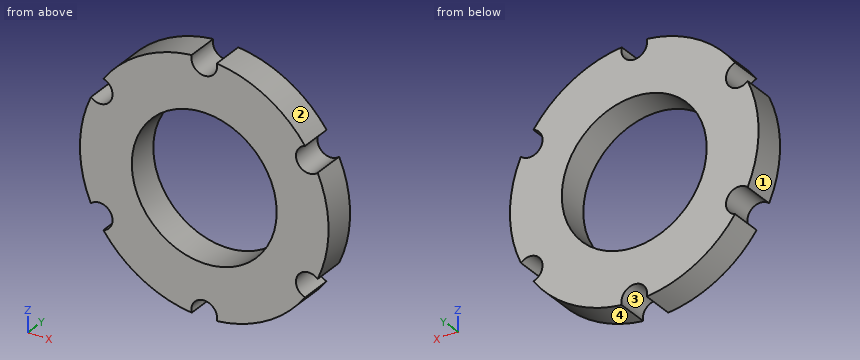
```python
from build123d import *

# Parameters (mm, degrees)
SKETCH1_R           = 30.861
SKETCH1_R_2         = 14.2875
BOSS_EXTRUDE1_DEPTH = 6.35
SKETCH2_R           = 2.54
CUT_EXTRUDE1_DEPTH  = 6.35
SKETCH3_R           = 30.861
SKETCH3_R_2         = 24.511
CUT_EXTRUDE2_DEPTH  = 45.103572894


with BuildPart() as part:
    # Sketch1 → Boss-Extrude1 (new body)
    with BuildSketch(Plane(origin=(0, 0, 0), x_dir=(1, 0, 0), z_dir=(0, 1, 0))):
        with Locations(Location((0, 0, 0), (0, 0, 270))):
            Circle(SKETCH1_R)
        with Locations(Location((0, 0, 0), (0, 0, 270))):
            Circle(SKETCH1_R_2, mode=Mode.SUBTRACT)
    extrude(amount=BOSS_EXTRUDE1_DEPTH)

    # Sketch2 → Cut-Extrude1 (cut)
    with BuildSketch(Plane(origin=(0, 6.35, 0), x_dir=(1, 0, 0), z_dir=(0, 1, 0))):
        with Locations(Location((0, 23.8125, 0), (0, 0, 270))):
            Circle(SKETCH2_R)
        with Locations(Location((0, -23.8125, 0), (0, 0, 270))):
            Circle(SKETCH2_R)
        with Locations(Location((20.622229928, 11.90625, 0), (0, 0, 270))):
            Circle(SKETCH2_R)
        with Locations(Location((20.622229928, -11.90625, 0), (0, 0, 270))):
            Circle(SKETCH2_R)
        with Locations(Location((-20.622229928, 11.90625, 0), (0, 0, 270))):
            Circle(SKETCH2_R)
        with Locations(Location((-20.622229928, -11.90625, 0), (0, 0, 270))):
            Circle(SKETCH2_R)
    extrude(amount=-CUT_EXTRUDE1_DEPTH, mode=Mode.SUBTRACT)

    # Sketch3 → Cut-Extrude2 (cut, through all)
    with BuildSketch(Plane(origin=(0, 6.35, 0), x_dir=(1, 0, 0), z_dir=(0, 1, 0))):
        Circle(SKETCH3_R)
        Circle(SKETCH3_R_2, mode=Mode.SUBTRACT)
    extrude(amount=-CUT_EXTRUDE2_DEPTH, mode=Mode.SUBTRACT)


solid = part.part
```
Input: part model. Units: mm. Frame: model coordinates. Face numbers are marked on the shaded views. Coordinates: 2 decimals unless noted, no trailing zeros. Loops run counter-clockwise (first coordinate to the right, second up) from the corner with the lowest first, then second, coordinate; pieces in that order, holes last.
Q1. Mould query, pull axis Z, two halves, no side actions, for the marked faces 1, 2, 3 and 4. Classes: +Z half, -Z half, draft (parallel to the pull), parting line (faces both ways), or undercut.
Results are:
face 1: parting line
face 2: +Z half
face 3: undercut
face 4: -Z half
Q2. Contact query for flat-ended pins moving along their axis: pin 1 (3 mm diameter, centred on y = 1.5, z = 18.5, fed in from +X); pin 2 (3 mm diameter, centred on y = 3.5, z = -11, fed in from -X); pin 3 (1.5 mm diameter, centred on x = -5, y = 4.5, fed in from +Z). Output: stop coordinate, or through.
Results are:
pin 1: stops at x = 17.66
pin 2: stops at x = -22.6
pin 3: stops at z = 24.14
Q3. Section C-C, the plane y = 1.25. Return the cut outline in (x, z) (1 decimal).
Results are:
outline: (-22.4, -10) arc R2.5 cw (long way) to (-19.9, -14.3) arc R24.5 ccw to (-2.5, -24.4) arc R2.5 cw (long way) to (2.5, -24.4) arc R24.5 ccw to (19.9, -14.3) arc R2.5 cw (long way) to (22.4, -10) arc R24.5 ccw to (22.4, 10) arc R2.5 cw (long way) to (19.9, 14.3) arc R24.5 ccw to (2.5, 24.4) arc R2.5 cw (long way) to (-2.5, 24.4) arc R24.5 ccw to (-19.9, 14.3) arc R2.5 cw (long way) to (-22.4, 10) arc R24.5 ccw to start; hole circle Ø28.6 at (0, 0)
Q4. Section D-D, the plane z = -16. Return the cut outline in (x, y), and give its area (3 significant figures).
Results are:
outline: (-18.57, 0) - (18.57, 0) - (18.57, 6.35) - (-18.57, 6.35) - close
area: 236 mm2
Q5. Line query: line 1 along X through (y, z) = (0.75, -7); line 2 along Z through (x, y) = (-8, 0.5); line 3 along X through (y, z) = (6.25, 2). Output: solid intervals per line, ascending.
Results are:
line 1: x = -23.49 to -12.46, 12.46 to 23.49
line 2: z = -23.17 to -11.84, 11.84 to 23.17
line 3: x = -24.43 to -14.15, 14.15 to 24.43
Q6. Section A-A, the plane x = 0. Return the cut outline in (y, z), and give its area (3 significant figures).
Results are:
outline: (0, -21.27) - (6.35, -21.27) - (6.35, -14.29) - (0, -14.29) - close; (0, 14.29) - (6.35, 14.29) - (6.35, 21.27) - (0, 21.27) - close
area: 88.7 mm2
Q7. Section B-B, the plane z = 0. Return the cut outline in (x, y).
Results are:
outline: (-24.51, 0) - (-14.29, 0) - (-14.29, 6.35) - (-24.51, 6.35) - close; (14.29, 0) - (24.51, 0) - (24.51, 6.35) - (14.29, 6.35) - close
